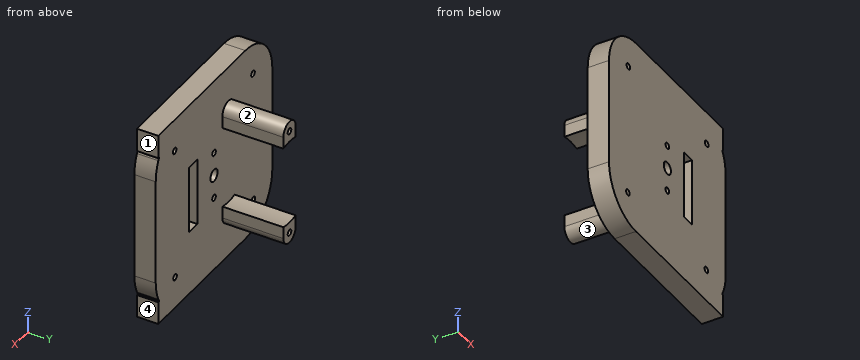
from build123d import *

# Parameters (mm, degrees)
SKETCH1_R           = 25.5
SKETCH1_R_2         = 1
SKETCH1_R_3         = 2
BOSS_EXTRUDE4_DEPTH = 7
SKETCH3_R           = 1
BOSS_EXTRUDE6_DEPTH = 20
SKETCH4_R           = 1
SKETCH4_W           = 4.52162884
SKETCH4_H           = 22.32
CUT_EXTRUDE2_DEPTH  = 10


with BuildPart() as part:
    # Sketch1 → Boss-Extrude4 (new body)
    with BuildSketch(Plane(origin=(0, 0, 0), x_dir=(1, 0, 0), z_dir=(0, 1, 0))):
        with BuildLine():
            Line((-23.098597486, 12.80927662), (-23.098597486, -22.19072338))
            ThreePointArc((-23.098597486, -22.19072338), (-18.705199204, -32.797325098), (-8.098597486, -37.19072338))
            Line((-8.098597486, -37.19072338), (40.463784198, -37.19072338))
            Line((40.463784198, -37.19072338), (40.463784198, -29.69072338))
            Line((40.463784198, -29.69072338), (40.167901675, -29.69072338))
            Line((40.167901675, -29.69072338), (40.167901675, -29.19072338))
            ThreePointArc((40.167901675, -29.19072338), (40.319108843, -28.896329756), (40.463784198, -28.598671807))
            ThreePointArc((40.463784198, -28.598671807), (41.53758585, -25.474339887), (41.901402514, -22.19072338))
            Line((41.901402514, -22.19072338), (41.901402514, 12.80927662))
            ThreePointArc((41.901402514, 12.80927662), (41.53758585, 16.092893127), (40.463784198, 19.217225047))
            ThreePointArc((40.463784198, 19.217225047), (40.319108843, 19.514882996), (40.167901675, 19.80927662))
            Line((40.167901675, 19.80927662), (40.167901675, 20.30927662))
            Line((40.167901675, 20.30927662), (40.463784198, 20.30927662))
            Line((40.463784198, 20.30927662), (40.463784198, 27.80927662))
            Line((40.463784198, 27.80927662), (-8.098597486, 27.80927662))
            ThreePointArc((-8.098597486, 27.80927662), (-18.705199204, 23.415878338), (-23.098597486, 12.80927662))
        make_face()
        with Locations((9.401402514, -4.69072338)):
            Circle(SKETCH1_R, mode=Mode.SUBTRACT)
        with Locations(Location((31.144043201, 17.278011972, 0), (0, 0, 270))):
            Circle(SKETCH1_R_2, mode=Mode.SUBTRACT)
        with Locations(Location((-12.567332839, 17.051917307, 0), (0, 0, 270))):
            Circle(SKETCH1_R_2, mode=Mode.SUBTRACT)
        with Locations(Location((-12.341238173, -26.659458733, 0), (0, 0, 270))):
            Circle(SKETCH1_R_2, mode=Mode.SUBTRACT)
        with Locations(Location((31.370137866, -26.433364067, 0), (0, 0, 270))):
            Circle(SKETCH1_R_2, mode=Mode.SUBTRACT)
        with Locations((9.401402514, -4.69072338)):
            Circle(SKETCH1_R)
        with Locations(Location((9.401402514, -4.69072338, 0), (0, 0, 270))):
            Circle(SKETCH1_R_3, mode=Mode.SUBTRACT)
    extrude(amount=BOSS_EXTRUDE4_DEPTH)

    # Sketch3 → Boss-Extrude6 (add)
    with BuildSketch(Plane(origin=(0, 7, 0), x_dir=(1, 0, 0), z_dir=(0, 1, 0))):
        with BuildLine():
            Line((-2.046619841, -18.234374208), (-2.046619841, -22.153505311))
            ThreePointArc((-2.046619841, -22.153505311), (1.353380159, -25.553505311), (4.753380159, -22.153505311))
            Line((4.753380159, -22.153505311), (4.753380159, -18.234374208))
            ThreePointArc((4.753380159, -18.234374208), (1.353380159, -18.653505311), (-2.046619841, -18.234374208))
        make_face()
        with Locations(Location((1.353380159, -22.153505311, 0), (0, 0, 270))):
            Circle(SKETCH3_R, mode=Mode.SUBTRACT)
        with BuildLine():
            Line((4.732675534, 8.927357463), (4.732675534, 12.846488565))
            ThreePointArc((4.732675534, 12.846488565), (1.332675534, 16.246488565), (-2.067324466, 12.846488565))
            Line((-2.067324466, 12.846488565), (-2.067324466, 8.927357463))
            ThreePointArc((-2.067324466, 8.927357463), (1.332675534, 9.346488565), (4.732675534, 8.927357463))
        make_face()
        with Locations(Location((1.332675534, 12.846488565, 0), (0, 0, 270))):
            Circle(SKETCH3_R, mode=Mode.SUBTRACT)
    extrude(amount=BOSS_EXTRUDE6_DEPTH)

    # Sketch4 → Cut-Extrude2 (cut)
    with BuildSketch(Plane.XZ):
        with Locations(Location((9.401402514, -3.05927662, 0), (0, 0, 270))):
            Circle(SKETCH4_R)
        with Locations(Location((9.401402514, 12.44072338, 0), (0, 0, 270))):
            Circle(SKETCH4_R)
        with Locations((20.980588094, 4.69072338)):
            Rectangle(SKETCH4_W, SKETCH4_H)
    extrude(amount=-CUT_EXTRUDE2_DEPTH, mode=Mode.SUBTRACT)


solid = part.part
Design review of the part built by this model. Coordinates are the model's own, in mm. Face numbers are marked on the shaded views. A direction names the side the tool comes from. Coordinates: 2 decimals unless noted, no trailing zeros. Order: outer loops, then holes, each group sorted by start corner. A loop starts at its lowest first (then second) coordinate and runs counter-clockwise, first axis right, second up. Notation, with made-up numbers: M 6,-29 L 28,-29 A17 ccw 28,2 Z; hole C -35.5,43.25 d2. An arc over 180 degrees is marked long. Use a Markdown table: item, result.
(1) Add section D-D (y = 5.25). Count the separate pieces of the cut face and the enclosed holes in it, then the cut area to 3 significant figures.
Worked answers:
| item | result |
|---|---|
| separate pieces | 1 |
| enclosed holes | 8 |
| area | 3,960 mm2 |
(2) Add section B-B (x = 19.5). Give the boundary of the cut face in (y, z).
Worked answers:
| item | result |
|---|---|
| outline | M 0,-27.81 L 7,-27.81 L 7,-6.47 L 0,-6.47 Z; M 0,15.85 L 7,15.85 L 7,37.19 L 0,37.19 Z |
(3) For P1, Ø8, axis at x = -7, y = 23.5, coming from the -Z side; P2, Ø1.5, axis at x = 12, z = 29, coming from the +Y side; P3, Ø5, axis at y = 21.5, z = 27.5, coming from the +X side; P4, Ø3, axis at x = 1.35, z = 22.15, coming from the +Y side, all flat-tipped, find the tip position at first contact; note any pin that passes through.
Worked answers:
| item | result |
|---|---|
| P1 | passes through |
| P2 | stops at y = 7 |
| P3 | stops at x = 3.21 |
| P4 | stops at y = 27 |
(4) For the marked faces 1, 2, 3 and 4, list the 3-axis set-ups (+Z, -Z, +X, -X, +Y, -Y) from which the entire face can be reached by the end or side of a thin tool; tool diameter is ignored.
Worked answers:
| item | result |
|---|---|
| face 1 | +Z, +X, +Y, -Y |
| face 2 | +Z, +Y |
| face 3 | -Z, +Y |
| face 4 | -Z, +X, +Y, -Y |
(5) Add section A-A (z = 14.5). Give the boundary of the cut face in (x, y).
Worked answers:
| item | result |
|---|---|
| outline | M -23.1,0 L 18.72,0 L 18.72,7 L -23.1,7 Z; M 23.24,0 L 41.9,0 L 41.9,7 L 23.24,7 Z |
(6) Wall thickness on probe 1 along Z at (x, y) = (2, 23.5); probe 2 along Y at (x, z) = (9, 27); probe 3 along Z at (x, y) = (-0.5, 12.75): over which ranges is each line inside the solid? List them lowest first.
Worked answers:
| item | result |
|---|---|
| probe 1 | z = -16.18 to -13.59, -12.1 to -9.33, 18.64 to 21.39, 22.92 to 25.49 |
| probe 2 | y = 0 to 7 |
| probe 3 | z = -15.71 to -9.23, 18.53 to 25 |
(7) Add section C-C (y = 12.25). Give the boundary of the cut face in (x, z), then the cut area to 3 significant figures.
Worked answers:
| item | result |
|---|---|
| outline | M -2.07,-12.85 A3.4 ccw 4.73,-12.85 L 4.73,-8.93 A14 cw -2.07,-8.93 Z; M -2.05,18.23 A14 cw 4.75,18.23 L 4.75,22.15 A3.4 ccw -2.05,22.15 Z; hole C 1.33,-12.85 d2; hole C 1.35,22.15 d2 |
| area | 79.5 mm2 |
